Autodesk Inventor part; units mm, degrees
ref_plane "YZ Plane" through (0, 0, 0) normal (1, 0, 0) x (0, 1, 0)
ref_plane "XZ Plane" through (0, 0, 0) normal (0, 1, 0) x (-1, 0, 0)
ref_plane "XY Plane" through (0, 0, 0) normal (0, 0, 1) x (1, 0, 0)
sketch "Sketch1" plane through (0, 0, 0) normal (1, 0, 0) x (0, 1, 0)
  line L0 (5.3982, 6.0675) -> (2.3982, 6.0675)
  line L1 (2.3982, 6.0675) -> (2.3982, -2.9325)
  line L2 (2.3982, -2.9325) -> (5.3982, -2.9325)
  line L3 (5.3982, -2.9325) -> (5.3982, 6.0675)
  point P0 (0, 0)
  dimension "d0" = 3
  dimension "d1" = 9
extrude "Extrusion1" add sketch "Sketch1" along normal mid plane 3
sketch "Sketch2" plane through (-1.5, 2.3982, 6.0675) normal (0, 0, 1) x (1, 0, 0)
  line L0 (0, 3) -> (3, 3)
  line L1 (0, 3) -> (0.5858, 3)
  line L2 (3, 3) -> (3, 0)
  line L3 (3, 0) -> (3, 0.5858)
  line L4 (1.2929, 2.7071) -> (2.7071, 1.2929)
  arc A0 (1.2929, 2.7071) -> (0.5858, 3) centre (0.5858, 2) ccw
  arc A1 (3, 0.5858) -> (2.7071, 1.2929) centre (2, 0.5858) ccw
  line L5 (0.5858, 3) -> (3, 3)
  arc A2 (1.2929, 2.7071) -> (0.5858, 3) centre (0.5858, 2) ccw
  arc A3 (3, 0.5858) -> (2.7071, 1.2929) centre (2, 0.5858) ccw
  line L6 (3, 3) -> (3, 0.5858)
  point P0 (1.5, -2.3982)
  point P1 (1, 3)
  point P2 (3, 1)
  dimension "d5" = 1
extrude "Extrusion2" cut sketch "Sketch2" against normal blind 50
sketch "Sketch4" plane through (-1.5, 0, 0) normal (-1, 0, 0) x (0, 0, 1)
  line L0 (6.0675, 5.3982) -> (-2.9325, 5.3982)
  line L1 (6.0675, 2.3982) -> (-2.9325, 2.3982)
  line L2 (6.0675, 3.6911) -> (-2.9325, 3.6911)
  line L3 (1.5675, 3.6911) -> (2.5531, 5.3982)
  line L4 (1.5675, 3.6911) -> (3.5387, 3.6911) construction
  line L5 (1.5675, 3.6911) -> (0.5819, 5.3982)
  line L6 (0.5819, 5.3982) -> (2.5531, 5.3982)
  point P0 (0, 0)
  dimension "d10" = 60
extrude "Extrusion3" cut sketch "Sketch4" against normal blind 50
sketch "Sketch5" plane through (-1.5, 2.3982, -2.9325) normal (0, -1, 0) x (1, 0, 0)
  line L0 (3, 9) -> (3, 0)
  line L1 (0, 0) -> (0, 9)
  line L2 (0, 6.75) -> (3, 6.75)
  line L3 (0, 2.25) -> (3, 2.25)
  line L4 (0, 2.25) -> (0, 6.75)
  line L5 (3, 2.25) -> (3, 6.75)
  point P0 (1.5, 2.9325)
  point P1 (0, 4.5)
extrude "Extrusion4" add sketch "Sketch5" along normal blind 7
sketch "Sketch7" plane through (-1.5, 0, 0) normal (-1, 0, 0) x (0, 0, 1)
  line L0 (-2.9325, 2.3982) -> (-0.6825, 2.3982)
  circle A0 centre (1.6026, -1.3518) radius 1
  point P0 (0.6868, -0.5794)
extrude "Extrusion5" cut sketch "Sketch7" against normal blind 3
thread "Thread1"
properties part number "Apoio móvel da ponte"
Input: part model. Units: mm. Frame: model coordinates. A direction names the side the tool comes from. Coordinates: 2 decimals unless noted, no trailing zeros. Loops run counter-clockwise (first coordinate to the right, second up) from the corner with the lowest first, then second, coordinate; pieces in that order, holes last.
(1) First-contact query: pin 1 Ø0.7 at (x, z) = (0, -2) entering from -Y; pin 2 Ø0.9 at (x, y) = (0, 0.5) entering from -Z. Flat tips, straight axial feed; report the tip coordinate or a pass-through.
(2) Section A-A on y = -2. Return the cut outline in (x, z), then the cut area to 3 significant figures.
(3) Section D-D on z = -0.5. Return the cut outline in (x, y), then the cut area to 3 significant figures.
(4) Set-up query: faces 1 (the face through (-0.47, 4.34, 1.94)), 2 (the face through (-0.02, -1.96, 0.81)), 3 (the face through (0, 2.398, -2)). Return all of +Z, -Z, +X, -X, +Y, -Y with unobstructed straight access to the full face (end or side cutting, diameter ignored); none if empty.
(5) Section C-C on x = 0.7. Return the cut outline in (y, z).
(6) Material intervals for probe 1 along Z at (x, y) = (-0.85, -3.5); probe 2 along Y at (x, z) = (-0.9, -1); probe 3 along Z at (x, y) = (-0.25, -1.25), sorted ascending.
(7) Pull-direction query (Z, two-part tool) for faces 4 (the face through (0, 2.398, 5)), 5 (the face through (-0.466, 4.343, 1.191)), 6 (the face through (0, 4, -2.932)), 7 (the face through (0, -1, 3.818)); classes: released by +Z, released by -Z, zero draft, split by the parting line, or undercut.
(8) Section B-B on z = 1. Return the cut outline in (x, y), then the cut area to 3 significant figures.
Data:
1. pin 1: stops at y = 2.4
1. pin 2: stops at z = -0.68
2. outline: (-1.5, -0.68) - (1.5, -0.68) - (1.5, 0.84) - (-1.5, 0.84) - close; (-1.5, 2.36) - (1.5, 2.36) - (1.5, 3.82) - (-1.5, 3.82) - close
2. area: 8.93 mm2
3. outline: (-1.5, -4.6) - (1.5, -4.6) - (1.5, 2.98) arc R1 ccw to (1.21, 3.69) - (-0.21, 5.11) arc R1 ccw to (-0.91, 5.4) - (-1.5, 5.4) - close
3. area: 28.0 mm2
4. face 1: +X, -X, +Y
4. face 2: +X, -X
4. face 3: -Z, +X, -X, -Y
5. outline: (-4.6, -0.68) - (2.4, -0.68) - (2.4, -2.93) - (4.2, -2.93) - (4.2, 1.27) - (3.69, 1.57) - (4.2, 1.86) - (4.2, 6.07) - (2.4, 6.07) - (2.4, 3.82) - (-4.6, 3.82) - close; hole circle Ø2 at (-1.35, 1.6)
6. probe 1: z = -0.68 to 3.82
6. probe 2: y = 2.4 to 5.4
6. probe 3: z = -0.68 to 0.61, 2.6 to 3.82
7. face 4: zero draft
7. face 5: undercut
7. face 6: released by -Z
7. face 7: released by +Z
8. outline: (-1.5, -4.6) - (1.5, -4.6) - (1.5, -2.15) - (-1.5, -2.15) - close; (-1.5, -0.55) - (1.5, -0.55) - (1.5, 2.98) arc R1 ccw to (1.21, 3.69) - (0.22, 4.67) - (-1.5, 4.67) - close
8. area: 22.2 mm2
